```python
from build123d import *

# Parameters (mm, degrees)
BOSS_EXTRUDE1_DEPTH = 50.8
SKETCH2_R           = 3.175
SKETCH2_W           = 6.35
SKETCH2_H           = 8.636
CUT_EXTRUDE1_DEPTH  = 56.811406764


with BuildPart() as part:
    # Sketch1 → Boss-Extrude1 (new body)
    with BuildSketch(Plane.XY):
        with BuildLine():
            Line((0, 0), (19.05, 0))
            ThreePointArc((19.05, 0), (20.6375, 5.924630657), (16.300369343, 1.5875))
            Line((16.300369343, 1.5875), (17.532203877, 2.2987))
            ThreePointArc((17.532203877, 2.2987), (19.9263, 4.692796123), (19.05, 1.4224))
            Line((19.05, 1.4224), (0, 1.4224))
            Line((0, 1.4224), (0, 0))
        make_face()
    extrude(amount=BOSS_EXTRUDE1_DEPTH)

    # Sketch2 → Cut-Extrude1 (cut, through all)
    with BuildSketch(Plane.XZ):
        with Locations(Location((6.985, 43.815, 0), (0, 0, 270))):
            Circle(SKETCH2_R)
        with Locations(Location((6.985, 6.985, 0), (0, 0, 270))):
            Circle(SKETCH2_R)
        with Locations((19.05, 46.482)):
            Rectangle(SKETCH2_W, SKETCH2_H)
        with Locations((19.05, 25.4)):
            Rectangle(SKETCH2_W, SKETCH2_H)
        with Locations((19.05, 4.318)):
            Rectangle(SKETCH2_W, SKETCH2_H)
    extrude(amount=-CUT_EXTRUDE1_DEPTH, mode=Mode.SUBTRACT)


solid = part.part
```
Check sheet for the modelled part. Datum: model origin and axes. Units: mm. A direction names the side the tool comes from. Give positions to 0.01 mm unless a question says otherwise; leave off trailing zeros. Loops run counter-clockwise (first coordinate to the right, second up) from the corner with the lowest first, then second, coordinate; pieces in that order, holes last. Notation, with made-up numbers: M 79,12.5 L 84,12.5 A27 ccw 84,44.5 Z; hole C 9.5,33.25 d8. An arc over 180 degrees is marked long. Answer in a Markdown table with one row per item.
1) Cross-section at A-A (y = 4.25). Enter the section's corners in (x, z), plus the area to 3 significant figures.
Solutions:
| item | result |
|---|---|
| outline | M 16.06,8.64 L 17.67,8.64 L 17.67,21.08 L 16.06,21.08 Z; M 16.06,29.72 L 17.67,29.72 L 17.67,42.16 L 16.06,42.16 Z; M 20.43,8.64 L 22.04,8.64 L 22.04,21.08 L 20.43,21.08 Z; M 20.43,29.72 L 22.04,29.72 L 22.04,42.16 L 20.43,42.16 Z |
| area | 79.8 mm^2 |
2) Thickness scan on line 1 (Z direction, x = 17, y = 4.75); line 2 (X direction, y = 3, z = 18.5); line 3 (Z direction, x = 4.75, y = 1.25). Record the ranges inside material, lowest first.
Solutions:
| item | result |
|---|---|
| line 1 | z = 8.64 to 21.08, 29.72 to 42.16 |
| line 2 | x = 15.88 to 17.31, 20.79 to 22.22 |
| line 3 | z = 0 to 4.73, 9.24 to 41.56, 46.07 to 50.8 |
3) Tool access check on faces 1 (the face through (10, 1.422, 25)), 2 (the face through (15.875, 1, 4)), 3 (the face through (15.875, 1, 46)), 4 (the face through (16.91, 1.94, 14.77)), 5 (the face through (15.875, 1, 25)). Record the directions out of +Z, -Z, +X, -X, +Y, -Y that give a thin tool (end or side, any length) a straight path to the whole face; none if there is none.
Solutions:
| item | result |
|---|---|
| face 1 | +Z, -Z, -X |
| face 2 | -Z, +X, +Y, -Y |
| face 3 | +Z, +X, +Y, -Y |
| face 4 | +Z, -Z |
| face 5 | +X, +Y, -Y |
4) Cross-section at D-D (x = 13.25). Enter the section's corners in (y, z).
Solutions:
| item | result |
|---|---|
| outline | M 0,0 L 1.42,0 L 1.42,50.8 L 0,50.8 Z |
5) Depth check by flat-ended pin: pin 1 (1.6 mm diameter, centred on y = 0.5, z = 3, fed in from +X) (3 decimals); pin 2 (3 mm diameter, centred on x = 19.05, y = 3.175, fed in from -Z); pin 3 (1.9 mm diameter, centred on x = 17.5, y = 3, fed in from +Z); pin 4 (2 mm diameter, centred on y = 4.5, z = 31.5, fed in from +X). Enter the tip coordinate at first touch or a pass-through.
Solutions:
| item | result |
|---|---|
| pin 1 | stops at x = 15.875 |
| pin 2 | passes through |
| pin 3 | stops at z = 42.16 |
| pin 4 | stops at x = 22.21 |
6) Mould release check, pull along Y, two halves, no side actions. Record for faces 6 (the face through (19.87, 4.724, 35.854)), 7 (the face through (9, 0, 25)), 8 (the face through (5.05, 0.7, 9.5)): released by +Y, released by -Y, zero draft, split by the parting line, or undercut.
Solutions:
| item | result |
|---|---|
| face 6 | undercut |
| face 7 | released by -Y |
| face 8 | zero draft |
7) Cross-section at B-B (x = 20). Enter the section's corners in (y, z).
Solutions:
| item | result |
|---|---|
| outline | M 0.15,8.64 L 1.7,8.64 L 1.7,21.08 L 0.15,21.08 Z; M 0.15,29.72 L 1.7,29.72 L 1.7,42.16 L 0.15,42.16 Z; M 4.65,8.64 L 6.2,8.64 L 6.2,21.08 L 4.65,21.08 Z; M 4.65,29.72 L 6.2,29.72 L 6.2,42.16 L 4.65,42.16 Z |
